Drawing for the job (mm, zero at the part's lowest x, y, z). Give positions to 0.01 mm unless a question says otherwise; leave off trailing zeros. Order: outer loops, then holes, each group sorted by start corner. A loop starts at its lowest first (then second) coordinate and runs counter-clockwise, first axis right, second up. Notation, with made-up numbers: (60.25, 38.25) -> (86.25, 38.25) arc R29 cw to (86.25, 65.25) -> close; hole circle Ø7 at (3.25, 42.25). An arc over 180 degrees is marked (long way). Use a Markdown table: item, result. Add a question column.
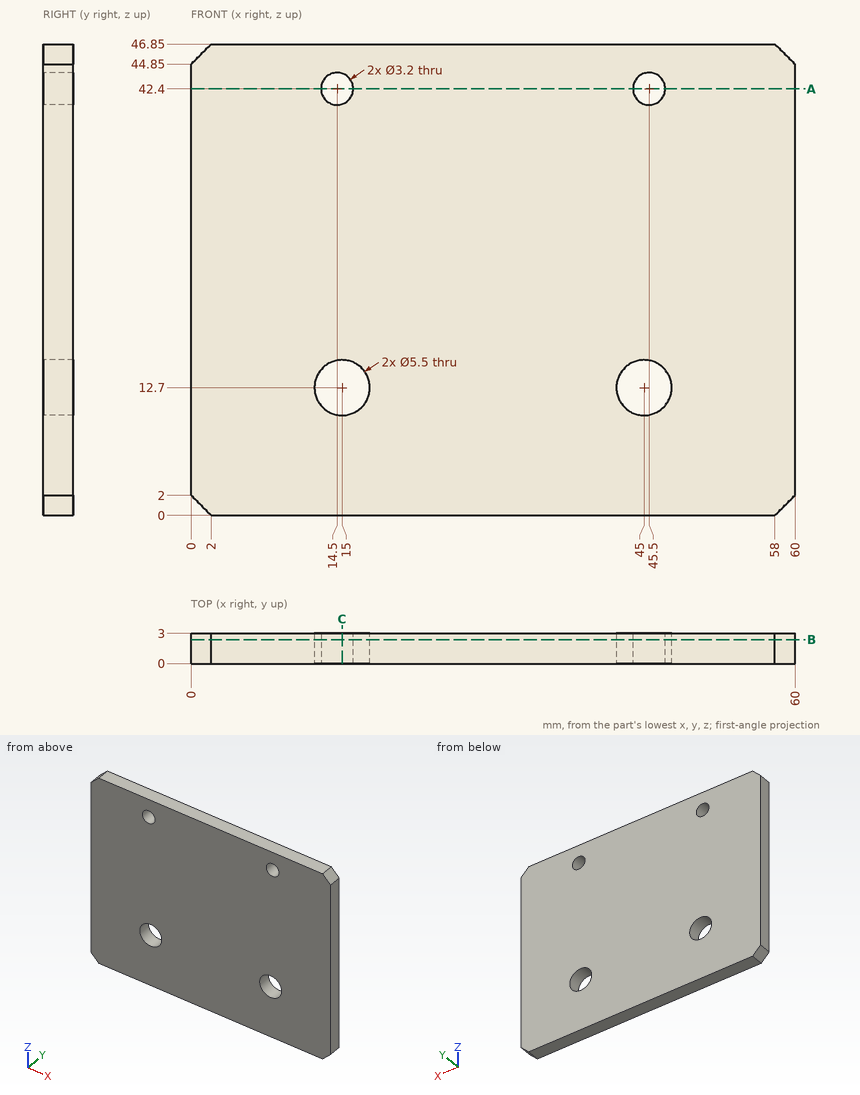
(1) Band-saw the part on C-C on x = 15. Give the cut face in (y, z), plus the area to 3 significant figures.
(2) Band-saw the part on A-A on z = 42.4. Give the cut face in (x, y).
(3) Wall check: probe 1 along X at (y, z) = (0.65, 12.5); probe 2 along X at (y, z) = (0.85, 41.5); probe 3 along Z at (x, y) = (45.5, 1.7). Give the ranges that are in metal, low to high.
(4) Band-saw the part on B-B on y = 2.4. Give the cut face in (x, z), plus the area to 3 significant figures.
Response:
| question | item | result |
|---|---|---|
| 1 | outline | (0, 0) -> (3, 0) -> (3, 9.95) -> (0, 9.95) -> close; (0, 15.45) -> (3, 15.45) -> (3, 40.88) -> (0, 40.88) -> close; (0, 43.92) -> (3, 43.92) -> (3, 46.85) -> (0, 46.85) -> close |
| 1 | area | 115 mm² |
| 2 | outline | (0, 0) -> (12.9, 0) -> (12.9, 3) -> (0, 3) -> close; (16.1, 0) -> (43.9, 0) -> (43.9, 3) -> (16.1, 3) -> close; (47.1, 0) -> (60, 0) -> (60, 3) -> (47.1, 3) -> close |
| 3 | probe 1 | x = 0 to 12.26, 17.74 to 42.26, 47.74 to 60 |
| 3 | probe 2 | x = 0 to 13.18, 15.82 to 44.18, 46.82 to 60 |
| 3 | probe 3 | z = 0 to 10, 15.4 to 40.8, 44 to 46.85 |
| 4 | outline | (0, 2) -> (2, 0) -> (58, 0) -> (60, 2) -> (60, 44.85) -> (58, 46.85) -> (2, 46.85) -> (0, 44.85) -> close; hole circle Ø5.5 at (15, 12.7); hole circle Ø3.2 at (14.5, 42.4); hole circle Ø5.5 at (45, 12.7); hole circle Ø3.2 at (45.5, 42.4) |
| 4 | area | 2,740 mm² |
